from build123d import *

# Parameters (mm, degrees)
F1_DEPTH      = 5.08
F1_DEPTH_BACK = 5.08
F2_R          = 25.4
F3_R          = 19.05
F4_DEPTH      = 25.4
F5_R          = 12.7
F6_DEPTH      = 25.4


with BuildPart() as f1:
    # F0 (on Right) → F1 (new body, two sides)
    with BuildSketch(Plane.YZ) as f1_sk:
        Polygon((30.48, 50.8), (-30.48, 50.8), (-58.42, -38.1), (58.42, -38.1), align=None)
    extrude(amount=F1_DEPTH)
    extrude(f1_sk.sketch, amount=-F1_DEPTH_BACK)

    # F2
    f2_edges = [f1.edges().sort_by_distance(p)[0] for p in [
        (0, -30.48, 50.8),
        (0, -58.42, -38.1),
        (0, 30.48, 50.8),
        (0, 58.42, -38.1),
    ]]
    fillet(f2_edges, radius=F2_R)

    # F3 (on face) → F4 (cut)
    with BuildSketch(Plane.YZ.offset(5.08)):
        with Locations((20.219197, 0)):
            Circle(F3_R)
    extrude(amount=-F4_DEPTH, mode=Mode.SUBTRACT)

    # F5 (on face) → F6 (cut)
    with BuildSketch(Plane.YZ.offset(5.08)):
        with Locations((-28.277963, -14.804346)):
            Circle(F5_R)
    extrude(amount=-F6_DEPTH, mode=Mode.SUBTRACT)


solid = f1.part
CAD build for the part. Positions are in the model's coordinates, mm. Round coordinates to 2 decimals unless told otherwise and drop trailing zeros. Order: outer loops, then holes, each group sorted by start corner. A loop starts at its lowest first (then second) coordinate and runs counter-clockwise, first axis right, second up. Notation, with made-up numbers: (-4, 58.5) - (17, 58.5) arc R12 cw to (17, 71.5) - close; hole circle Ø3 at (-7, 63.5). An arc over 180 degrees is marked (long way). Return JSON: item names as keys, results as strings.
(1) Cut at C-C (z = 2.5). Give the cut face in (x, y), then the cut area to 3 significant figures.
Answer key:
{"outline": "(-5.08, -45.66) - (5.08, -45.66) - (5.08, 1.33) - (-5.08, 1.33) - close; (-5.08, 39.1) - (5.08, 39.1) - (5.08, 45.66) - (-5.08, 45.66) - close", "area": "544 mm^2"}
(2) Wall check: probe 1 along Y at (x, z) = (-1.75, -3.5); probe 2 along Z at (x, y) = (4.5, 26); probe 3 along Z at (x, y) = (-2, 25). Give the ranges that are in metal, low to high. Write a range as from..to.
Answer key:
{"probe 1": "y = -47.55..-34.07, -22.49..1.49, 38.94..47.55", "probe 2": "z = -38.01..-18.15, 18.15..46.49", "probe 3": "z = -38.07..-18.44, 18.44..47.12"}
(3) Pull direction Y, two halves, no side cores. Call faces 1 (the face through (0.071, -41.973, 14.232)), 2 (the face through (5.08, -1, 7)), 3 (the face through (0.07, 38.39, 5.72)): +Y half, -Y half, draft (parallel to the pull), parting line (faces both ways), or undercut.
Answer key:
{"face 1": "-Y half", "face 2": "draft", "face 3": "undercut"}
(4) Cut at D-D (z = 31.5). Give the cut face in (x, y).
Answer key:
{"outline": "(-5.08, -36.55) - (5.08, -36.55) - (5.08, 36.55) - (-5.08, 36.55) - close"}
(5) Cut at A-A (z = -23). Give the cut face in (x, y), then the cut area to 3 significant figures.
Answer key:
{"outline": "(-5.08, -47.03) - (5.08, -47.03) - (5.08, -37.98) - (-5.08, -37.98) - close; (-5.08, -18.58) - (5.08, -18.58) - (5.08, 47.03) - (-5.08, 47.03) - close", "area": "759 mm^2"}
(6) Cut at B-B (x = -3). Give the cut face in (y, z), then the cut area to 3 significant figures.
Answer key:
{"outline": "(-48.04, -5.08) arc R25.4 ccw to (-23.81, -38.1) - (23.81, -38.1) arc R25.4 ccw to (48.04, -5.08) - (36.07, 33.02) arc R25.4 ccw to (11.84, 50.8) - (-11.84, 50.8) arc R25.4 ccw to (-36.07, 33.02) - close; hole circle Ø25.4 at (-28.28, -14.8); hole circle Ø38.1 at (20.22, 0)", "area": "5,580 mm^2"}
(7) Pin check, flat tips, straight feed: pin 1 Ø3 at (x, y) = (-0.5, 24.5) entering from +Z; pin 2 Ø3 at (x, z) = (0.5, -18.5) entering from +Y; pin 3 Ø1 at (x, z) = (3.5, 37) entering from -Y. Stop position of each tip, or through.
Answer key:
{"pin 1": "stops at z = 48.22", "pin 2": "stops at y = 48.85", "pin 3": "stops at y = -34.68"}
